The model under review builds one solid part; all positions refer to its coordinate system, in mm. Face numbers are marked on the shaded views. A direction names the side the tool comes from. Coordinates: 2 decimals unless noted, no trailing zeros. Order: outer loops, then holes, each group sorted by start corner. A loop starts at its lowest first (then second) coordinate and runs counter-clockwise, first axis right, second up.
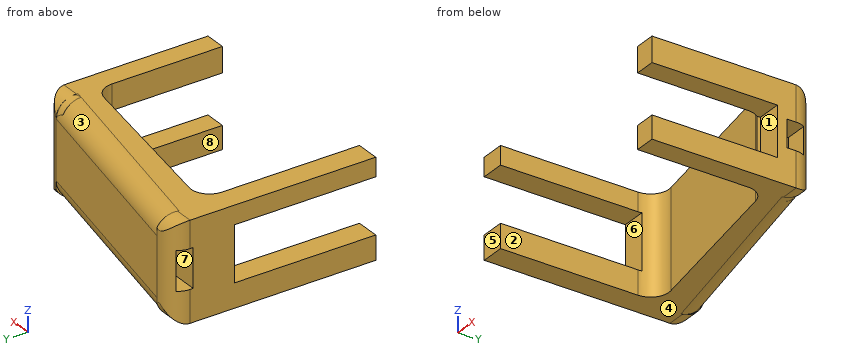
from build123d import *

# Parameters (mm, degrees)
SALIENTE_EXTRUIR1_DEPTH = 800
CROQUIS2_W              = 450.891954089
CROQUIS2_H              = 1153.204494417
CORTAR_EXTRUIR1_DEPTH   = 479
CROQUIS6_W              = 1733.666634621
CROQUIS6_H              = 800
CORTAR_EXTRUIR4_DEPTH   = 1
REDONDEO1_R             = 160
CORTAR_EXTRUIR5_DEPTH   = 204
CORTAR_EXTRUIR6_DEPTH   = 204
CROQUIS9_W              = 1543.706277585
CROQUIS9_H              = 195.894282261
CORTAR_EXTRUIR7_DEPTH   = 73
CROQUIS10_W             = 406.798125856
CROQUIS10_H             = 1024.288303457
CORTAR_EXTRUIR8_DEPTH   = 204
CROQUIS11_W             = 316.726975088
CROQUIS11_H             = 118.414803419
CORTAR_EXTRUIR9_DEPTH   = 204
CROQUIS13_W             = 222.696577042
CROQUIS13_H             = 152.562571667
CORTAR_EXTRUIR10_DEPTH  = 204


with BuildPart() as part:
    # Croquis1 → Saliente-Extruir1 (new body)
    with BuildSketch(Plane.XY):
        with BuildLine():
            Line((0, 0), (0, 1517.029414592))
            ThreePointArc((0, 1517.029414592), (54.901664159, 1633.030735793), (179.417420271, 1664.116515946))
            Line((179.417420271, 1664.116515946), (1879.417420271, 1324.116515946))
            ThreePointArc((1879.417420271, 1324.116515946), (1966.001321201, 1272.127750433), (2000, 1177.029414592))
            Line((2000, 1177.029414592), (2000, 0))
            Line((2000, 0), (1827.655470466, 0))
            Line((1827.655470466, 0), (1827.655470466, 903.590756555))
            ThreePointArc((1827.655470466, 903.590756555), (1792.016786618, 1000.655113392), (1702.035612225, 1051.596191212))
            Line((1702.035612225, 1051.596191212), (368.421499763, 1271.275294141))
            ThreePointArc((368.421499763, 1271.275294141), (246.977001167, 1237.631175636), (194.041358004, 1123.269859484))
            Line((194.041358004, 1123.269859484), (194.041358004, 0))
            Line((194.041358004, 0), (0, 0))
        make_face()
    extrude(amount=SALIENTE_EXTRUIR1_DEPTH)

    # Croquis2 → Cortar-Extruir1 (cut)
    with BuildSketch(Plane.ZY):
        with Locations((422.175014136, 576.602247208)):
            Rectangle(CROQUIS2_W, CROQUIS2_H)
    extrude(amount=-CORTAR_EXTRUIR1_DEPTH, mode=Mode.SUBTRACT)

    # Croquis6 → Cortar-Extruir4 (cut)
    with BuildSketch(Plane(origin=(326.923076923, 1634.615384615, 0), x_dir=(0.9805806756909202, -0.19611613513818404, 0), z_dir=(0.19611613513818404, 0.9805806756909202, 0))):
        with Locations((716.406472984, -400)):
            Rectangle(CROQUIS6_W, CROQUIS6_H)
    extrude(amount=-CORTAR_EXTRUIR4_DEPTH, mode=Mode.SUBTRACT)

    # Redondeo1
    redondeo1_edges = [part.edges().sort_by_distance(p)[0] for p in [
        (1029.221304136, 1493.13593527, 0),
        (1029.221304136, 1493.13593527, 800),
    ]]
    fillet(redondeo1_edges, radius=REDONDEO1_R)

    # Croquis7 → Cortar-Extruir5 (cut)
    with BuildSketch(Plane.ZY):
        with BuildLine():
            Line((0, 1517.029414592), (0, 1667.029414592))
            Line((0, 1667.029414592), (136.758196867, 1667.029414592))
            ThreePointArc((136.758196867, 1667.029414592), (39.321568117, 1618.521784269), (0, 1517.029414592))
        make_face()
        with BuildLine():
            ThreePointArc((800, 1517.029414592), (772.596251195, 1607.268062357), (699.64037564, 1667.029414592))
            Line((699.64037564, 1667.029414592), (800, 1667.029414592))
            Line((800, 1667.029414592), (800, 1517.029414592))
        make_face()
    extrude(amount=-CORTAR_EXTRUIR5_DEPTH, mode=Mode.SUBTRACT)

    # Croquis8 → Cortar-Extruir6 (cut)
    with BuildSketch(Plane(origin=(2000, 0, 0), x_dir=(0, 0, -1), z_dir=(1, 0, 0))):
        with BuildLine():
            ThreePointArc((-640, 1324.116515946), (-748.667630167, 1281.75735047), (-800, 1177.029414592))
            Line((-800, 1177.029414592), (-800, 1324.116515946))
            Line((-800, 1324.116515946), (-640, 1324.116515946))
        make_face()
        with BuildLine():
            ThreePointArc((0, 1177.029414592), (-25.457205923, 1264.264892498), (-93.837620587, 1324.116515946))
            Line((-93.837620587, 1324.116515946), (0, 1324.116515946))
            Line((0, 1324.116515946), (0, 1177.029414592))
        make_face()
    extrude(amount=-CORTAR_EXTRUIR6_DEPTH, mode=Mode.SUBTRACT)

    # Croquis9 → Cortar-Extruir7 (cut)
    with BuildSketch(Plane(origin=(297.309540517, 1486.547702586, 0), x_dir=(0.9805806756909202, -0.19611613513818407, 0), z_dir=(0.19611613513818407, 0.9805806756909202, 0))):
        with Locations((770.502378662, -401.181328028)):
            Rectangle(CROQUIS9_W, CROQUIS9_H)
    extrude(amount=-CORTAR_EXTRUIR7_DEPTH, mode=Mode.SUBTRACT)

    # Croquis10 → Cortar-Extruir8 (cut)
    with BuildSketch(Plane(origin=(2000, 0, 0), x_dir=(0, 0, -1), z_dir=(1, 0, 0))):
        with Locations((-391.027888744, 512.144151728)):
            Rectangle(CROQUIS10_W, CROQUIS10_H)
    extrude(amount=-CORTAR_EXTRUIR8_DEPTH, mode=Mode.SUBTRACT)

    # Croquis11 → Cortar-Extruir9 (cut)
    with BuildSketch(Plane.ZY):
        with Locations((420.951887064, 1550.388466328)):
            Rectangle(CROQUIS11_W, CROQUIS11_H)
    extrude(amount=-CORTAR_EXTRUIR9_DEPTH, mode=Mode.SUBTRACT)

    # Croquis13 → Cortar-Extruir10 (cut)
    with BuildSketch(Plane(origin=(2000, 0, 0), x_dir=(0, 0, -1), z_dir=(1, 0, 0))):
        with Locations((-400, 1177.029414592)):
            Rectangle(CROQUIS13_W, CROQUIS13_H)
    extrude(amount=-CORTAR_EXTRUIR10_DEPTH, mode=Mode.SUBTRACT)


solid = part.part
(1) Consider section A-A (y = 214.5). Give the boundary of the cut face in (x, z), then the cut area to 3 significant figures.
(2) Consider section D-D (y = 972.5). Give the boundary of the cut face in (x, z).
(3) The part is to be moulded in two halves that separate along Z. For the marked faces 1, 2 and 3, say which applies: +Z half, -Z half, draft (parallel to the pull), parting line (faces both ways), or undercut.
(4) Consider section B-B (z = 329). Give the boundary of the cut face in (x, y).
(5) Wall thickness on line 1 (Z direction, x = 997.5, y = 1307); line 2 (X direction, y = 906, z = 135.5); line 3 (Y direction, x = 110.5, z = 509): over which ranges is each line inside the solid? List them lowest first.
(6) Consider section C-C (z = 552.5). Give the boundary of the cut face in (x, y), then the cut area to 3 significant figures.
(7) Insertion check: pin 1 Ø1.8 at (x, z) = (1799, 92.5) entering from -Y; pin 2 Ø3 at (x, z) = (1483, 568) entering from -Y; pin 3 Ø5 at (x, z) = (1576, 291) entering from +Y. Each pin has a flat end and moves straight along its axis. Give the tip position at first contact, or say it passes through.
(8) Tool access review of the marked faces 4, 5, 6, 7 and 8: name each direction out of +Z, -Z, +X, -X, +Y, -Y from which nothing blocks a thin tool from reaching the whole face with its end or side.
Findings:
1. outline: (0, 0) - (194.04, 0) - (194.04, 196.73) - (0, 196.73) - close; (0, 647.62) - (194.04, 647.62) - (194.04, 800) - (0, 800) - close; (1827.66, 0) - (2000, 0) - (2000, 187.63) - (1827.66, 187.63) - close; (1827.66, 594.43) - (2000, 594.43) - (2000, 800) - (1827.66, 800) - close
1. area: 136,000 mm2
2. outline: (0, 0) - (194.04, 0) - (194.04, 196.73) - (0, 196.73) - close; (0, 647.62) - (194.04, 647.62) - (194.04, 800) - (0, 800) - close; (1810.89, 0) - (2000, 0) - (2000, 187.63) - (1810.89, 187.63) - close; (1810.89, 594.43) - (2000, 594.43) - (2000, 800) - (1810.89, 800) - close
3. face 1: undercut
3. face 2: draft
3. face 3: +Z half
4. outline: (0, 1153.2) - (197.06, 1153.2) arc R150 cw to (368.42, 1271.28) - (1702.04, 1051.6) arc R150 cw to (1796, 995.76) - (1796, 1024.29) - (2000, 1024.29) - (2000, 1100.75) - (1796, 1100.75) - (1796, 1115.5) - (1795.4, 1112.48) - (281.67, 1415.23) - (295.99, 1486.81) - (1796, 1186.81) - (1796, 1253.31) - (1979.16, 1253.31) arc R150 ccw to (1879.42, 1324.12) - (1879.22, 1323.14) - (179.22, 1663.14) - (179.42, 1664.12) arc R150 ccw to (31.97, 1609.6) - (204, 1609.6) - (204, 1491.18) - (0, 1491.18) - close
5. line 1: z = 0 to 303.23, 499.13 to 800
5. line 2: x = 0 to 194.04, 1827.64 to 2000
5. line 3: y = 1153.2 to 1491.18, 1609.6 to 1661.74
6. outline: (0, 1153.2) - (197.06, 1153.2) arc R150 cw to (368.42, 1271.28) - (1702.04, 1051.6) arc R150 cw to (1796, 995.76) - (1796, 1024.29) - (2000, 1024.29) - (2000, 1177.03) arc R150 ccw to (1879.42, 1324.12) - (1879.22, 1323.14) - (179.22, 1663.14) - (179.42, 1664.12) arc R150 ccw to (31.97, 1609.6) - (204, 1609.6) - (204, 1491.18) - (0, 1491.18) - close
6. area: 669,000 mm2
7. pin 1: stops at y = 990.52
7. pin 2: stops at y = 1087.43
7. pin 3: stops at y = 1384.28
8. face 4: -Z, +X, -X, +Y, -Y
8. face 5: +Z, -Z, +X, -X, -Y
8. face 6: -X, -Y
8. face 7: -X
8. face 8: +Z, -Z, -Y
